```python
from build123d import *

# Parameters (mm, degrees)
F0_W        = 160
F0_H        = 74
F1_DEPTH    = 2
F2_W        = 97.5
F2_H        = 40
F2_R        = 4.5
F2_R_2      = 3.5
F3_DEPTH    = 2
F4_W        = 9
F4_H        = 9
F5_DEPTH    = 10
F6_R        = 1.75
F7_DEPTH    = 8
F8_W        = 160
F8_H        = 74
F9_DEPTH    = 12
F9_FACE_W   = 160
F9_FACE_H   = 74
F9_FACE_W_2 = 154
F9_FACE_H_2 = 68
F10_ANGLE   = 45
F11_W       = 25
F11_H       = 4
F12_DEPTH   = 3
F13_R       = 2
F14_R       = 4


# Not quite as in the source:
# - a feature names something its author has since deleted; it is built from what else it names


with BuildPart() as f1:
    # F0 (on Top) → F1 (new body)
    with BuildSketch(Plane.XY):
        Rectangle(F0_W, F0_H)
    extrude(amount=F1_DEPTH)

    # F2 (on face) → F3 (cut)
    with BuildSketch(Plane.XY.offset(2)):
        with Locations((12.25, -2)):
            Rectangle(F2_W, F2_H)
        with Locations((-62.5, 2)):
            Circle(F2_R)
        with Locations((-62.5, -15)):
            Circle(F2_R_2)
    extrude(amount=-F3_DEPTH, mode=Mode.SUBTRACT)

    # F4 (on face) → F5 (join)
    with BuildSketch(Plane.XY.offset(2)):
        with Locations((72.5, 29.5)):
            Rectangle(F4_W, F4_H)
        with Locations((-72.5, 29.5)):
            Rectangle(F4_W, F4_H)
        with Locations((-72.5, -20.5)):
            Rectangle(F4_W, F4_H)
        with Locations((72.5, -20.5)):
            Rectangle(F4_W, F4_H)
    extrude(amount=F5_DEPTH)

    # F6 (on face) → F7 (cut)
    with BuildSketch(Plane.XY.offset(12)):
        with Locations((-72.5096613169, 29.5301117003)):
            Circle(F6_R)
        with Locations((-72.5096613169, -20.5968357623)):
            Circle(F6_R)
        with Locations((72.5096613169, 29.5301117003)):
            Circle(F6_R)
        with Locations((72.5096613169, -20.5968357623)):
            Circle(F6_R)
    extrude(amount=-F7_DEPTH, mode=Mode.SUBTRACT)

    # F8 (on face) → F9 (join)
    with BuildSketch(Plane.XY.offset(2)):
        Rectangle(F8_W, F8_H)
        Polygon((-77, 25), (-77, 34), (-68, 34), (68, 34), (77, 34), (77, 25), (77, -16), (77, -25), (77, -34), (-77, -34), (-77, -25), (-77, -16), align=None, mode=Mode.SUBTRACT)
    extrude(amount=F9_DEPTH)

    # F9_face (on face) → F10 (revolve)
    with BuildSketch(Plane.XY.offset(14)):
        Rectangle(F9_FACE_W, F9_FACE_H)
        Rectangle(F9_FACE_W_2, F9_FACE_H_2, mode=Mode.SUBTRACT)
    revolve(axis=Axis((0, 37, 14), (-1, 0, 0)), revolution_arc=F10_ANGLE)

    # F11 (on face) → F12 (cut)
    with BuildSketch(Plane.YZ.offset(80)):
        with Locations((-2.5, 15)):
            Rectangle(F11_W, F11_H)
    extrude(amount=-F12_DEPTH, mode=Mode.SUBTRACT)

    # F13
    f13_edges = [f1.edges().sort_by_distance(p)[0] for p in [
        (80, 37, 7),
        (80, -31.367085, 42.318574),
        (80, -37, 7),
        (-80, 37, 7),
        (-80, -31.367085, 42.318574),
        (-80, -37, 7),
        (-77, 34.228361, 15.14805),
        (77, 34.228361, 15.14805),
    ]]
    fillet(f13_edges, radius=F13_R)

    # F14
    f14_edges = [f1.edges().sort_by_distance(p)[0] for p in [
        (-77, -28.595447, 41.170524),
        (77, -28.595447, 41.170524),
    ]]
    fillet(f14_edges, radius=F14_R)


solid = f1.part
```
Work out the finished part from the listing and answer in its coordinate system (mm). A direction names the side the tool comes from. Give positions to 0.01 mm unless a question says otherwise; leave off trailing zeros. Loops run counter-clockwise (first coordinate to the right, second up) from the corner with the lowest first, then second, coordinate; pieces in that order, holes last. Notation, with made-up numbers: (-7, 31.5) -> (38, 31.5) arc R13 ccw to (38, 47.5) -> close; hole circle Ø8 at (2.5, 32). An arc over 180 degrees is marked (long way). Write item = value, one per line. Start each with the question number.
(1) Find section C-C on y = -7. Give the vertices of the cut face in (x, z).
(2) Find section D-D on y = 2. Give the vertices of the cut face in (x, z).
(3) Find section A-A on x = 22.5. Give the vertices of the cut face in (y, z).
(4) Find the intervals of material crossed by probe 1 along Y at (x, z) = (49.5, 9); probe 2 along X at (y, z) = (-15.5, 44.5); probe 3 along Z at (x, y) = (72, -2.5), in increasing order. Write a range as from..to.
(5) The mould has two halves that part along Z. Classify faces 1 (the flat face through (72, -16, 7)), 2 (the cylindrical face through (1.092, -31.522, 41.942)), 3 (the flat face through (68, 29, 7)): +Z half, -Z half, draft (parallel to the pull), parting line (faces both ways), or undercut.
(6) Which of the six approach directions +Z, -Z, +X, -X, +Y, -Y give full straight-line access (tool end or side, diameter ignored) to faces 4 (the cylindrical face through (-66, -15, 1)), 5 (the flat face through (-77, -5, 26)), 6 (the flat face through (79, 10, 15)), 7 (the flat face through (-73, 25, 7))?
(7) Given pin 1 Ø6 at (x, y) = (-53, -7.5) entering from +Z; pin 2 Ø2.5 at (x, y) = (78, 3) entering from -Z; pin 3 Ø3.5 at (x, y) = (78.5, -8.5) entering from +Z; pin 4 Ø1 at (x, y) = (72, -21) entering from +Z, each flat-ended and moving along its own axis, determine where each tip first touches the part or whether it passes through.
(8) Find section B-B on x = -62.5. Give the vertices of the cut face in (y, z), and give its area (3 significant figures).
From the geometry:
q1.outline = (-80, 0) -> (-36.5, 0) -> (-36.5, 2) -> (-77, 2) -> (-77, 58) -> (-80, 58) -> close; (61, 0) -> (80, 0) -> (80, 13) -> (77, 13) -> (77, 2) -> (61, 2) -> close; (77, 17) -> (80, 17) -> (80, 58) -> (77, 58) -> close
q2.outline = (-80, 0) -> (-67, 0) -> (-67, 2) -> (-77, 2) -> (-77, 49) -> (-80, 49) -> close; (-58, 0) -> (-36.5, 0) -> (-36.5, 2) -> (-58, 2) -> close; (61, 0) -> (80, 0) -> (80, 13) -> (77, 13) -> (77, 2) -> (61, 2) -> close; (77, 17) -> (80, 17) -> (80, 49) -> (77, 49) -> close
q3.outline = (-37, 0) -> (-22, 0) -> (-22, 2) -> (-34, 2) -> (-34, 14) arc R71 cw to (-13.2, 64.2) -> (-15.33, 66.33) arc R74 ccw to (-37, 14) -> close; (18, 0) -> (37, 0) -> (37, 14) -> (34.88, 16.12) arc R3 ccw to (34, 14) -> (34, 2) -> (18, 2) -> close
q4.probe_1 = -37..-34, 34..37
q4.probe_2 = -80..-77, 77..80
q4.probe_3 = 0..2
q5.face_1 = undercut
q5.face_2 = +Z half
q5.face_3 = draft
q6.face_4 = -Z
q6.face_5 = none
q6.face_6 = +X
q6.face_7 = +Z
q7.pin_1 = 2
q7.pin_2 = 0
q7.pin_3 = 61.25
q7.pin_4 = 60.58
q8.outline = (-37, 0) -> (-18.5, 0) -> (-18.5, 2) -> (-34, 2) -> (-34, 14) arc R71 cw to (-13.2, 64.2) -> (-15.33, 66.33) arc R74 ccw to (-37, 14) -> close; (-11.5, 0) -> (-2.5, 0) -> (-2.5, 2) -> (-11.5, 2) -> close; (6.5, 0) -> (37, 0) -> (37, 14) -> (34.88, 16.12) arc R3 ccw to (34, 14) -> (34, 2) -> (6.5, 2) -> close
q8.area = 362 mm^2
